Part model, mm, in its own coordinate system. Face numbers are marked on the shaded views. Round coordinates to 2 decimals unless told otherwise and drop trailing zeros. Loops run counter-clockwise (first coordinate to the right, second up) from the corner with the lowest first, then second, coordinate; pieces in that order, holes last. Notation, with made-up numbers: M 27,-20 L 31,-20 A7 cw 31,-12 Z; hole C 75.5,17.25 d9. An arc over 180 degrees is marked long. Put each result on its own line as item: value. Start each with the question number.
1) Slice it at B-B on z = 0. Give the cut face in (x, y).
2) Slice it at A-A on y = 0. Give the cut face in (x, z).
3) Drop flat-ended pins along their axis: pin 1 Ø1 at (x, y) = (-2.5, 2.5) entering from -Z; pin 2 Ø1 at (x, y) = (-2.5, 0.5) entering from -Z; pin 3 Ø1.2 at (x, z) = (0, 0) entering from +Y; pin 4 Ø1.5 at (x, z) = (1.5, 2) entering from -Y. Give the stop position or say it passes through.
4) Slice it at C-C on x = 0. Give the cut face in (y, z), then the cut area to 3 significant figures.
5) Probe line 1 along Z through (x, y) = (1.5, 0); line 2 along X through (y, z) = (2.5, 2); line 3 along Z through (x, y) = (1, 2.5). List the from-to ranges inside material, lowest first.
6) Pull direction Y, two halves, no side cores. Call the marked faces 1, 2 and 3: +Y half, -Y half, draft (parallel to the pull), parting line (faces both ways), or undercut.
7) Slice it at D-D on y = -1.5. Give the cut face in (x, z).
```python
from build123d import *

# Parameters (mm, degrees)
F1_ANGLE = 270
F14_T    = -0.75
F3_D     = 2
F5_D     = 2
F7_ANGLE = 135
F9_D     = 2
F11_D    = 2
F13_D    = 2


with BuildPart() as f1:
    # F0 (on Top) → F1 (revolve)
    with BuildSketch(Plane.XY):
        with BuildLine():
            ThreePointArc((4.5, 0), (0, 4.5), (-4.5, 0))
            Line((-4.5, 0), (4.5, 0))
        make_face()
    revolve(axis=Axis((0.171331, 0, 0), (1, 0, 0)), revolution_arc=F1_ANGLE)

    # F14
    f14_openings = [f1.faces().sort_by_distance(p)[0] for p in [
        (0, 1.909859, 0),
        (0, 0, -1.909859),
    ]]
    offset(amount=F14_T, openings=f14_openings)

    # F3 (through all)
    with Locations(Plane.YZ):
        with Locations((0, 0)):
            Hole(F3_D / 2)

    # F5 (through all)
    with Locations(Plane(origin=(0, 0, 0), x_dir=(0, 1, 0), z_dir=(-1, 0, 0))):
        with Locations((0, 0)):
            Hole(F5_D / 2)


with BuildPart() as f1_1:
    # F7: moved
    add(f1.part.rotate(Axis((0, 0, 0), (-1, 0, 0)), F7_ANGLE))

    # F9 (through all)
    with Locations(Plane.XZ):
        with Locations((0, 0)):
            Hole(F9_D / 2)

    # F11 (through all)
    with Locations(Plane.XY):
        with Locations((0, 0)):
            Hole(F11_D / 2)

    # F13 (through all)
    with Locations(Plane(origin=(0, 0, 0), x_dir=(1, 0, 0), z_dir=(0, 0, -1))):
        with Locations((0, 0)):
            Hole(F13_D / 2)


solid = f1_1.part
```
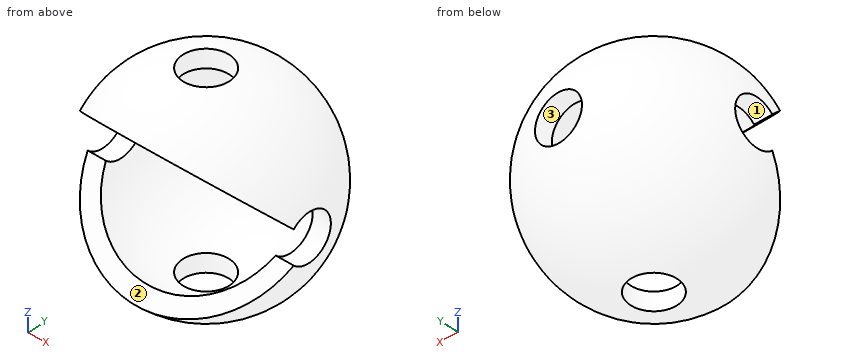
Recorded:
1. outline: M -4.39,1 L -3.61,1 A3.75 cw -1,3.61 L -1,4.39 A4.5 ccw Z; M 1,3.61 A3.75 cw 3.61,1 L 4.39,1 A4.5 ccw 1,4.39 Z
2. outline: M -4.39,-1 A4.5 ccw -1,-4.39 L -1,-3.61 A3.75 cw -3.61,-1 Z; M -4.39,1 L -3.61,1 A3.75 cw -1,3.61 L -1,4.39 A4.5 ccw Z; M 1,-4.39 A4.5 ccw 4.39,-1 L 3.61,-1 A3.75 cw 1,-3.61 Z; M 1,3.61 A3.75 cw 3.61,1 L 4.39,1 A4.5 ccw 1,4.39 Z
3. pin 1: stops at z = -3.32
3. pin 2: stops at z = -4.01
3. pin 3: passes through
3. pin 4: stops at y = -2.75
4. outline: M -3.18,-3.18 A4.5 ccw -1,-4.39 L -1,-3.61 A3.75 cw -2.65,-2.65 Z; M -3.18,3.18 L -2.65,2.65 A3.75 cw -1,3.61 L -1,4.39 A4.5 ccw Z; M 1,-4.39 A4.5 ccw 4.39,-1 L 3.61,-1 A3.75 cw 1,-3.61 Z; M 1,3.61 A3.75 cw 3.61,1 L 4.39,1 A4.5 ccw 1,4.39 Z
4. area: 10.0 mm2
5. line 1: z = -4.24 to -3.44, 3.44 to 4.24
5. line 2: x = -3.16 to -1.95, 1.95 to 3.16
5. line 3: z = -3.61 to -2.61, 2.61 to 3.61
6. face 1: undercut
6. face 2: -Y half
6. face 3: draft
7. outline: M -3.97,-1.5 A4.24 ccw 3.97,-1.5 L 3.09,-1.5 A3.44 cw -3.09,-1.5 Z; M -3.97,1.5 L -3.09,1.5 A3.44 cw 3.09,1.5 L 3.97,1.5 A4.24 ccw Z
